Verification items for the finished model (mm, model axes). A direction names the side the tool comes from. Round coordinates to 2 decimals unless told otherwise and drop trailing zeros. Order: outer loops, then holes, each group sorted by start corner. A loop starts at its lowest first (then second) coordinate and runs counter-clockwise, first axis right, second up. Notation, with made-up numbers: M -7.75,17 L 1.25,17 A17 cw 1.25,34 Z; hole C 83,1.25 d10. An arc over 180 degrees is marked long. Use CSV: the item, a comma, the result in double quotes. Start each with the question number.
Q1. Sectioned sample at C-C (y = -7). Enter the section's corners in (x, z), and give its area (3 significant figures).
Q2. Sectioned sample at B-B (y = 20). State how many separate pieces and enclosed holes the cut face has, and give its area (3 significant figures).
Q3. Gauge pin test, flat ends, axial feed: pin 1 Ø9 at (x, y) = (-27, 7) entering from -Z; pin 2 Ø16 at (x, y) = (10, 10.5) entering from -Z. Record the tip position at first contact, or that the pin passes through.
Q4. Scan lines: line 1 (Y direction, x = -15.5, z = 3.55); line 2 (X direction, y = 20, z = 4.65); line 3 (Y direction, x = 16.25, z = 4.7). Record each from-to range of solid material in increasing order.
Q5. Set-up check for faces 1 (the face through (39, 24.2, 2.5)), 2 (the face through (27, -7, 2)): record each of +Z, -Z, +X, -X, +Y, -Y from which the full face is reachable in a straight line by a thin tool's end or side.
Q6. Sectioned sample at D-D (x = 37.5). Enter the section's corners in (y, z), and give its area (3 significant figures).
Q7. Sectioned sample at A-A (x = 4). Enter the section's corners in (y, z).
Q8. Mould release check, pull along X, two halves, no side actions. Record for faces 3 (the face through (-27, 0, 0)), 4 (the face through (-19.776, -2.483, 4.704)), 5 (the face through (-40, 0, 2)): +X half, -X half, draft (parallel to the pull), parting line (faces both ways), or undercut.
Autodesk Inventor part; units mm, degrees
ref_plane "YZ Plane" through (0, 0, 0) normal (1, 0, 0) x (0, 1, 0)
ref_plane "XZ Plane" through (0, 0, 0) normal (0, 1, 0) x (-1, 0, 0)
ref_plane "XY Plane" through (0, 0, 0) normal (0, 0, 1) x (1, 0, 0)
sketch "Skizze1" plane through (0, 0, 0) normal (0, 0, 1) x (1, 0, 0)
  line L0 (-40, 35) -> (40, 35)
  line L1 (40, 35) -> (40, -35)
  line L2 (40, -35) -> (-40, -35)
  line L3 (-40, -35) -> (-40, 35)
  line L4 (-40, 35) -> (40, -35) construction
  line L5 (40, 35) -> (-40, -35) construction
  point P0 (0, 0)
  dimension "d0" = 80
  dimension "d1" = 70
extrude "Extrusion1" add sketch "Skizze1" along normal blind 5
sketch "Skizze2" plane through (0, 0, 5) normal (0, 0, 1) x (1, 0, 0)
  line L0 (-37.5, 25) -> (37.5, 25)
  line L1 (37.5, 25) -> (37.5, -20)
  line L2 (37.5, -20) -> (-37.5, -20)
  line L3 (-37.5, -20) -> (-37.5, 25)
  line L4 (-40, 35) -> (-40, -35)
  line L5 (40, -35) -> (40, 35)
  line L6 (-40, -35) -> (40, -35)
  point P0 (0, 0)
  dimension "d4" = 2.5
  dimension "d5" = 2.5
  dimension "d6" = 15
  dimension "d7" = 60
hole "Bohrung1" at (-37.5, 25, 5) at (37.5, 25, 5) at (37.5, -20, 5) at (-37.5, -20, 5) direction (0, 0, -1) diameter 3.4 end through all
sketch "Skizze3" plane through (0, 0, 5) normal (0, 0, 1) x (1, 0, 0)
  line L0 (-25, -30) -> (25, -30)
  line L1 (-40, 35) -> (-40, -35)
  line L2 (40, -35) -> (40, 35)
  line L3 (-40, -35) -> (40, -35)
  point P0 (0, 0)
  dimension "d15" = 15
  dimension "d16" = 15
  dimension "d17" = 5
hole "Bohrung2" at (-25, -30, 5) at (25, -30, 5) direction (0, 0, -1) diameter 4.5 end through all
sketch "Skizze4" plane through (0, 0, 5) normal (0, 0, 1) x (1, 0, 0)
  line L0 (-13.15, 24.8) -> (13.15, 24.8)
  line L1 (13.75, 24.2) -> (13.75, 17.7)
  line L2 (11.25, 15.2) -> (-11.25, 15.2)
  line L3 (-13.75, 17.7) -> (-13.75, 24.2)
  line L4 (-13.75, 24.8) -> (13.75, 15.2) construction
  line L5 (13.75, 24.8) -> (-13.75, 15.2) construction
  line L6 (40, 35) -> (-40, 35)
  arc A0 (-13.15, 24.8) -> (-13.75, 24.2) centre (-13.15, 24.2) ccw
  arc A1 (13.75, 24.2) -> (13.15, 24.8) centre (13.15, 24.2) ccw
  arc A2 (-13.75, 17.7) -> (-11.25, 15.2) centre (-11.25, 17.7) ccw
  arc A3 (11.25, 15.2) -> (13.75, 17.7) centre (11.25, 17.7) ccw
  line L7 (48.751, 18.7264) -> (89.4803, 18.7264) construction
  line L8 (89.4803, 18.7264) -> (89.4803, 14.9967) construction
  line L9 (89.4803, 14.9967) -> (48.751, 14.9967) construction
  line L10 (48.751, 14.9967) -> (48.751, 18.7264) construction
  line L11 (-17.198, -1.3) -> (17.198, -1.3)
  line L12 (21.25, -1.3) -> (21.25, -1.3)
  line L13 (16.3869, -12.7) -> (-16.3869, -12.7)
  line L14 (-21.25, -1.3) -> (-21.25, -1.3)
  line L15 (-21.25, -1.3) -> (21.25, -12.7) construction
  line L16 (21.25, -1.3) -> (-21.25, -12.7) construction
  line L17 (-40, -35) -> (40, -35)
  line L18 (-20.5464, -5.2904) -> (-19.7353, -9.8904)
  line L19 (20.5464, -5.2904) -> (19.7353, -9.8904)
  arc A4 (-17.198, -1.3) -> (-20.5464, -5.2904) centre (-17.198, -4.7) ccw
  arc A5 (20.5464, -5.2904) -> (17.198, -1.3) centre (17.198, -4.7) ccw
  arc A6 (-19.7353, -9.8904) -> (-16.3869, -12.7) centre (-16.3869, -9.3) ccw
  arc A7 (16.3869, -12.7) -> (19.7353, -9.8904) centre (16.3869, -9.3) ccw
  line L20 (50.079, -7.9738) -> (119.9486, -7.9738) construction
  line L21 (119.9486, -7.9738) -> (119.9486, -12.597) construction
  line L22 (119.9486, -12.597) -> (50.079, -12.597) construction
  line L23 (50.079, -12.597) -> (50.079, -7.9738) construction
  line L24 (40, -35) -> (40, 35)
  point P0 (0, 0)
  point P1 (0, 20)
  point P2 (0, 20)
  point P3 (0, -7)
  point P4 (0, -7)
  point P5 (0, -7)
  point P6 (-19.2399, -12.7)
  point P7 (19.2399, -12.7)
  dimension "d25" = 27.5
  dimension "d26" = 9.6
  dimension "d28" = 0.6
  dimension "d29" = 2.5
  dimension "d32" = 15
  dimension "d49" = 28
  dimension "d50" = 11.4
  dimension "d51" = 42.5
  dimension "d52" = 80
  dimension "d53" = 19.2399
  dimension "d54" = 19.2399
  dimension "d55" = 80
  dimension "d56" = 3.4
  dimension "d64" = 26.25
extrude "Extrusion2" cut sketch "Skizze4" against normal through all
sketch "Skizze5" plane through (0, 0, 5) normal (0, 0, 1) x (1, 0, 0)
  line L0 (40, 35) -> (-40, 35)
  line L1 (0, -7) -> (23.5, -7)
  line L2 (0, -7) -> (-23.5, -7)
  line L3 (-40, -35) -> (40, -35)
  line L4 (-13.75, 17.7) -> (-13.75, 24.2)
  line L5 (13.75, 24.2) -> (13.75, 17.7)
  point P0 (0, 0)
  point P1 (-16.25, 20)
  point P2 (16.25, 20)
  dimension "d57" = 28
  dimension "d58" = 23.5
  dimension "d59" = 23.5
  dimension "d65" = 15
  dimension "d66" = 2.5
  dimension "d67" = 2.5
hole "Bohrung3" at (-23.5, -7, 5) at (23.5, -7, 5) at (-16.25, 20, 5) at (16.25, 20, 5) direction (0, 0, -1) diameter 3.1 end through all
sketch "Skizze6" plane through (0, 0, 0) normal (0, 0, -1) x (-1, 0, 0)
  line L0 (40, 35) -> (-40, 35)
  line L1 (-26.4, -0.25) -> (26.4, -0.25)
  line L2 (27, -0.85) -> (27, -13.15)
  line L3 (26.4, -13.75) -> (-26.4, -13.75)
  line L4 (-27, -13.15) -> (-27, -0.85)
  line L5 (-27, -0.25) -> (27, -13.75) construction
  line L6 (27, -0.25) -> (-27, -13.75) construction
  line L7 (-40, -35) -> (40, -35)
  arc A0 (-26.4, -0.25) -> (-27, -0.85) centre (-26.4, -0.85) ccw
  arc A1 (27, -0.85) -> (26.4, -0.25) centre (26.4, -0.85) ccw
  arc A2 (26.4, -13.75) -> (27, -13.15) centre (26.4, -13.15) ccw
  arc A3 (-27, -13.15) -> (-26.4, -13.75) centre (-26.4, -13.15) ccw
  circle A4 centre (-16.25, 20) radius 1.55
  line L8 (-16.25, 20) -> (16.6724, 20)
  line L9 (13.15, 24.8) -> (-13.15, 24.8)
  line L10 (0, 24.8) -> (0, 15.2)
  line L11 (11.25, 15.2) -> (-11.25, 15.2)
  line L12 (-18.4, 25.5) -> (18.4, 25.5)
  line L13 (19, 24.9) -> (19, 15.1)
  line L14 (18.4, 14.5) -> (-18.4, 14.5)
  line L15 (-19, 15.1) -> (-19, 24.9)
  line L16 (-19, 25.5) -> (19, 14.5) construction
  line L17 (19, 25.5) -> (-19, 14.5) construction
  arc A5 (-18.4, 25.5) -> (-19, 24.9) centre (-18.4, 24.9) ccw
  arc A6 (19, 24.9) -> (18.4, 25.5) centre (18.4, 24.9) ccw
  arc A7 (18.4, 14.5) -> (19, 15.1) centre (18.4, 15.1) ccw
  arc A8 (-19, 15.1) -> (-18.4, 14.5) centre (-18.4, 15.1) ccw
  point P0 (0, 0)
  point P1 (0, -7)
  point P2 (0, -7)
  point P3 (0, 20)
  dimension "d60" = 28
  dimension "d61" = 13.5
  dimension "d62" = 54
  dimension "d63" = 0.6
  dimension "d68" = 11
  dimension "d69" = 38
  dimension "d70" = 0.6
extrude "Extrusion3" cut sketch "Skizze6" against normal blind 4.4
sketch "Skizze7" plane through (0, 0, 0) normal (0, 0, -1) x (-1, 0, 0)
  line L0 (40, -35) -> (40, 35)
  line L1 (40, 35) -> (-40, 35)
  point P0 (0, 0)
  point P1 (27, 20)
hole "Bohrung4" at (-27, 20, 0) direction (0, 0, 1) diameter 11 end through all
sketch "Skizze10" plane through (0, 0, 0) normal (0, 0, -1) x (-1, 0, 0)
  line L0 (40, 35) -> (-40, 35)
  point P0 (0, 0)
  point P1 (-23.5, 20)
  dimension "d84" = 15
  dimension "d85" = 23.5
hole "Bohrung5" at (23.5, 20, 0) direction (0, 0, 1) diameter 3.1 end through all counterbore diameter 3.5 counterbore depth 2.5
sketch "Skizze11" plane through (0, 0, 0) normal (0, 0, -1) x (-1, 0, 0)
  line L0 (40, -35) -> (40, 35)
  line L1 (40, 35) -> (-40, 35)
  point P0 (0, 0)
  point P1 (27, 7)
  dimension "d93" = 13
  dimension "d94" = 28
hole "Bohrung6" at (-27, 7, 0) direction (0, 0, 1) diameter 11 depth 4
sketch "Skizze12" plane through (0, 0, 0) normal (0, 0, -1) x (-1, 0, 0)
  arc A0 (-27, -13.15) -> (-26.4, -13.75) centre (-26.4, -13.15) ccw
  line L0 (-40, -35) -> (40, -35)
  line L1 (-33, 14.5) -> (17, 14.5)
  line L2 (19, 12.5) -> (19, 1.75)
  line L3 (17, -0.25) -> (-33, -0.25)
  line L4 (-35, 1.75) -> (-35, 12.5)
  arc A1 (-35, 1.75) -> (-33, -0.25) centre (-33, 1.75) ccw
  arc A2 (17, -0.25) -> (19, 1.75) centre (17, 1.75) ccw
  arc A3 (-33, 14.5) -> (-35, 12.5) centre (-33, 12.5) ccw
  circle A4 centre (-16.25, 20) radius 1.55
  line L5 (-40, 35) -> (-40, -35)
  line L6 (-33, -13.75) -> (33, -13.75)
  line L7 (35, -15.75) -> (35, -23)
  line L8 (33, -25) -> (-33, -25)
  line L9 (-35, -23) -> (-35, -15.75)
  arc A5 (-33, -13.75) -> (-35, -15.75) centre (-33, -15.75) ccw
  arc A6 (-35, -23) -> (-33, -25) centre (-33, -23) ccw
  arc A7 (33, -25) -> (35, -23) centre (33, -23) ccw
  arc A8 (35, -15.75) -> (33, -13.75) centre (33, -15.75) ccw
  line L10 (40, -35) -> (40, 35)
  arc A9 (19, 12.5) -> (17, 14.5) centre (17, 12.5) ccw
  point P0 (0, 0)
  point P1 (27, -13.15)
  point P2 (19, 14.5)
  point P3 (-27, -0.85)
  point P4 (13.75, 17.7)
  point P5 (-11.25, 15.2)
  point P6 (19, 15.1)
  point P7 (-26.4, -0.25)
  point P8 (18.4, 14.5)
  dimension "d106" = 2
  dimension "d107" = 2
  dimension "d111" = 5
  dimension "d112" = 2
  dimension "d113" = 10
  dimension "d114" = 5
  dimension "d115" = 2
extrude "Extrusion4" cut sketch "Skizze12" against normal blind 3 contours L1 A9 L2 A2 L3 A1 L4 A3 | L6 A8 L7 A7 L8 A6 L9 A5
properties part number "Rückwand_DVI"
Verdict:
1,outline,"M -40,0 L -27,0 L -27,4.4 L -25.05,4.4 L -25.05,5 L -40,5 Z; M -21.95,4.4 L -20.24,4.4 L -20.24,5 L -21.95,5 Z; M 20.24,4.4 L 21.95,4.4 L 21.95,5 L 20.24,5 Z; M 25.05,4.4 L 27,4.4 L 27,0 L 40,0 L 40,5 L 25.05,5 Z"
1,area,"134 mm²"
2,separate pieces,"6"
2,enclosed holes,"0"
2,area,"141 mm²"
3,pin 1,"stops at z = 4"
3,pin 2,"stops at z = 3"
4,line 1,"y = -35 to -13.75, -0.25 to 14.5, 25.5 to 35"
4,line 2,"x = -40 to -32.5, -21.5 to -17.8, -14.7 to -13.75, 13.75 to 14.7, 17.8 to 21.95, 25.05 to 40"
4,line 3,"y = -35 to -12.7, -1.3 to 18.45, 21.55 to 35"
5,face 1,"+Z, -Z"
5,face 2,"-Z"
6,outline,"M -35,0 L -21.7,0 L -21.7,5 L -35,5 Z; M -18.3,0 L 23.3,0 L 23.3,5 L -18.3,5 Z; M 26.7,0 L 35,0 L 35,5 L 26.7,5 Z"
6,area,"316 mm²"
7,outline,"M -35,0 L -25,0 L -25,3 L -13.75,3 L -13.75,4.4 L -12.7,4.4 L -12.7,5 L -35,5 Z; M -1.3,4.4 L -0.25,4.4 L -0.25,3 L 14.5,3 L 14.5,4.4 L 15.2,4.4 L 15.2,5 L -1.3,5 Z; M 24.8,4.4 L 25.5,4.4 L 25.5,0 L 35,0 L 35,5 L 24.8,5 Z"
8,face 3,"draft"
8,face 4,"undercut"
8,face 5,"-X half"
